For this review, take the finished solid that the model builds, in its own axes (mm). Face numbers are marked on the shaded views. A direction names the side the tool comes from. Coordinates: 2 decimals unless noted, no trailing zeros. Loops run counter-clockwise (first coordinate to the right, second up) from the corner with the lowest first, then second, coordinate; pieces in that order, holes last. Notation, with made-up numbers: (87.5, 35) - (93.5, 35) arc R22 cw to (93.5, 47) - close; hole circle Ø11 at (12.5, 40). An arc over 180 degrees is marked (long way). Use one line per item in the form item = value. Start each with the question number.
1. Add section C-C on y = 5.75. Give the boundary of the cut face in (x, z), and give its area (3 significant figures).
2. Add section B-B on x = 0. Give the boundary of the cut face in (y, z) (3 decimals), and give its area (3 significant figures).
3. Add section D-D on y = 18.5. Give the boundary of the cut face in (x, z) (3 decimals).
4. Draft analysis for pull direction X (two halves, no side actions). For the marked faces 3, 4 and 5, state which applies: +X half, -X half, draft (parallel to the pull), parting line (faces both ways), or undercut.
5. To check wall thickness, follow probe 1 along X at (y, z) = (6.75, 0); probe 2 along X at (y, z) = (13.9, 0); probe 3 along Y at (x, z) = (-2, -10.5). State the ranges of each line that lie inside material, in increasing order.
6. Add section A-A on z = 0. Give the boundary of the cut face in (x, y) (3 decimals).
7. Machinability: for the marked faces 1 and 2, which of the approach directions +Z, -Z, +X, -X, +Y, -Y give a long, thin tool a straight path to every point of the face, cutting with its end or side? Answer none if there is none.
8. For pin 1 Ø6.5 at (x, z) = (0.5, 1.5) entering from +Y; pin 2 Ø3.5 at (x, z) = (11.03, 11.41) entering from -Y; pin 3 Ø2 at (x, z) = (-11.03, -11.41) entering from +Y; pin 4 Ø1.5 at (x, z) = (-13, -2) entering from +Y, all flat-tipped, find the tip position at first contact; note any pin that passes through.
```python
from build123d import *

# Parameters (mm, degrees)
CUT_EXTRUDE2_DEPTH        = 38.909021354
CUT_EXTRUDE2_DEPTH_BACK   = 38.909021354
SKETCH4_OUTSIDE_W         = 52.124
SKETCH4_OUTSIDE_H         = 52.124
SKETCH4_OUTSIDE_W_2       = 33.02
SKETCH4_OUTSIDE_H_2       = 33.02
F_6_32_TAPPED_HOLE2_D     = 2.7051
F_6_32_TAPPED_HOLE2_DEPTH = 9.398
F_6_32_TAPPED_HOLE2_TIP   = 0.81269403
FILLET1_R                 = 1.016


with BuildPart() as part:
    # Vent Valve Body Profile → Revolve2 (revolve)
    with BuildSketch(Plane.XY, mode=Mode.PRIVATE) as revolve2_sk:
        Polygon((-19.05, 26.67), (-19.05, 0), (-4.445, 0), (-4.445, 3.302), (-2.794, 3.302), (-2.794, 12.954), (-6.477, 12.954), (-6.477, 14.986), (-13.335, 14.986), (-13.335, 26.67), align=None)
    revolve(revolve2_sk.sketch.rotate(Axis((0, 11.135829036, 0), (0, -1, 0)), 270), axis=Axis((0, 11.135829036, 0), (0, -1, 0)))

    # Sketch4 outside → Cut-Extrude2 (cut, two sides: drawn at the far end of the back side and taken through both)
    with BuildSketch(Plane(origin=(0, 26.67, 0), x_dir=(1, 0, 0), z_dir=(0, 1, 0)).offset(-CUT_EXTRUDE2_DEPTH_BACK)):
        Rectangle(SKETCH4_OUTSIDE_W, SKETCH4_OUTSIDE_H)
        Rectangle(SKETCH4_OUTSIDE_W_2, SKETCH4_OUTSIDE_H_2, mode=Mode.SUBTRACT)
    extrude(amount=CUT_EXTRUDE2_DEPTH + CUT_EXTRUDE2_DEPTH_BACK, mode=Mode.SUBTRACT)

    # #6-32 Tapped Hole2
    with Locations(Plane(origin=(0, 26.67, 0), x_dir=(1, 0, 0), z_dir=(0, 1, 0))):
        with Locations((11.032567234, 11.414818668), (11.032567234, -11.414818668), (-11.032567234, -11.414818668), (-11.032567234, 11.414818668)):
            Hole(F_6_32_TAPPED_HOLE2_D / 2, depth=F_6_32_TAPPED_HOLE2_DEPTH)
            with Locations((0, 0, -(F_6_32_TAPPED_HOLE2_DEPTH + F_6_32_TAPPED_HOLE2_TIP / 2))):  # 118° drill point
                Cone(0, F_6_32_TAPPED_HOLE2_D / 2, F_6_32_TAPPED_HOLE2_TIP, mode=Mode.SUBTRACT)

    # Fillet1
    fillet1_edges = [part.edges().sort_by_distance(p)[0] for p in [
        (0, 26.67, -13.335),
    ]]
    fillet(fillet1_edges, radius=FILLET1_R)


solid = part.part
```
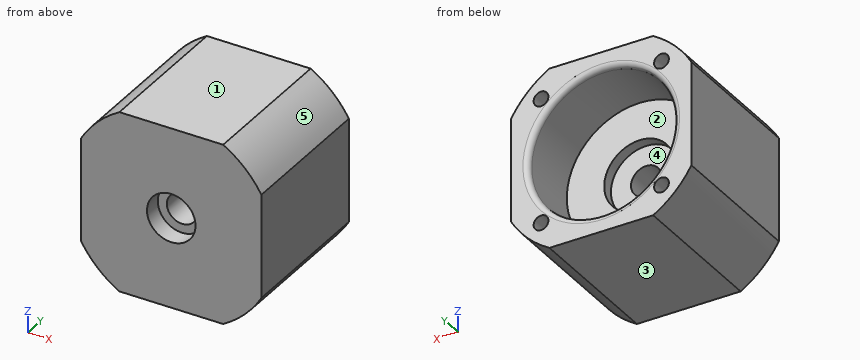
Conclusion:
q1.outline = (-16.51, -9.5) arc R19.05 ccw to (-9.5, -16.51) - (9.5, -16.51) arc R19.05 ccw to (16.51, -9.5) - (16.51, 9.5) arc R19.05 ccw to (9.5, 16.51) - (-9.5, 16.51) arc R19.05 ccw to (-16.51, 9.5) - close; hole circle Ø5.59 at (0, 0)
q1.area = 985 mm^2
q2.outline = (0, -16.51) - (26.67, -16.51) - (26.67, -14.351) arc R1.016 ccw to (25.654, -13.335) - (14.986, -13.335) - (14.986, -6.477) - (12.954, -6.477) - (12.954, -2.794) - (3.302, -2.794) - (3.302, -4.445) - (0, -4.445) - close; (0, 4.445) - (3.302, 4.445) - (3.302, 2.794) - (12.954, 2.794) - (12.954, 6.477) - (14.986, 6.477) - (14.986, 13.335) - (25.654, 13.335) arc R1.016 ccw to (26.67, 14.351) - (26.67, 16.51) - (0, 16.51) - close
q2.area = 459 mm^2
q3.outline = (-16.51, -9.504) arc R19.05 ccw to (-9.504, -16.51) - (9.504, -16.51) arc R19.05 ccw to (16.51, -9.504) - (16.51, 9.504) arc R19.05 ccw to (9.504, 16.51) - (-9.504, 16.51) arc R19.05 ccw to (-16.51, 9.504) - close; hole circle Ø26.67 at (0, 0); hole circle Ø2.705 at (-11.033, -11.415); hole circle Ø2.705 at (-11.033, 11.415); hole circle Ø2.705 at (11.033, -11.415); hole circle Ø2.705 at (11.033, 11.415)
q4.face_3 = draft
q4.face_4 = undercut
q4.face_5 = +X half
q5.probe_1 = -16.51 to -2.79, 2.79 to 16.51
q5.probe_2 = -16.51 to -6.48, 6.48 to 16.51
q5.probe_3 = 0 to 14.99
q6.outline = (-16.51, 0) - (-4.445, 0) - (-4.445, 3.302) - (-2.794, 3.302) - (-2.794, 12.954) - (-6.477, 12.954) - (-6.477, 14.986) - (-13.335, 14.986) - (-13.335, 25.654) arc R1.016 ccw to (-14.351, 26.67) - (-16.51, 26.67) - close; (2.794, 3.302) - (4.445, 3.302) - (4.445, 0) - (16.51, 0) - (16.51, 26.67) - (14.351, 26.67) arc R1.016 ccw to (13.335, 25.654) - (13.335, 14.986) - (6.477, 14.986) - (6.477, 12.954) - (2.794, 12.954) - close
q7.face_1 = +Z, +X, -X, +Y, -Y
q7.face_2 = +Y
q8.pin_1 = 12.95
q8.pin_2 = 0
q8.pin_3 = 17.06
q8.pin_4 = 26.57
